Here's how the part is built. I have some questions about the finished solid (model axes, mm). A direction names the side the tool comes from. Coordinates: 2 decimals unless noted, no trailing zeros. Loops run counter-clockwise (first coordinate to the right, second up) from the corner with the lowest first, then second, coordinate; pieces in that order, holes last.
from build123d import *

# Parameters (mm, degrees)
F0_R     = 6.7
F0_R_2   = 4.1
F1_DEPTH = 2
F2_R     = 6.2
F2_R_2   = 4.1
F3_DEPTH = 10
F4_SIZE  = 0.5


with BuildPart() as f1:
    # F0 (on Top) → F1 (new body)
    with BuildSketch(Plane.XY):
        Circle(F0_R)
        Circle(F0_R_2, mode=Mode.SUBTRACT)
    extrude(amount=F1_DEPTH)

    # F2 (on face) → F3 (join)
    with BuildSketch(Plane.XY.offset(2)):
        Circle(F2_R)
        Circle(F2_R_2, mode=Mode.SUBTRACT)
    extrude(amount=F3_DEPTH)

    # F4
    f4_edges = [f1.edges().sort_by_distance(p)[0] for p in [
        (-4.1, 0, 12),
        (-6.2, 0, 12),
    ]]
    chamfer(f4_edges, length=F4_SIZE)


solid = f1.part
Q1. Will these pins go through, and if not, where does the flat tip stop? P1, Ø2, axis at x = -5, z = 6, coming from the +Y side; P2, Ø1, axis at y = 3.5, z = 8, coming from the -X side; P3, Ø5, axis at y = -0.5, z = 9, coming from the +X side.
Q2. We'd pull the mould along Y, two halves only. Please class faces 3 (the cylindrical face through (-0.534, 4.065, 5.67)), 4 (the cylindrical face through (-6.694, 0.295, 0.986)), 5 (the flat face through (-4, 3, 12)): pulls with the +Y half, pulls with the -Y half, needs draft (parallel to the pull), parting line crosses it, or undercut.
Q3. Please list where these lines run through material, in increasing order: probe 1 along Y at (x, z) = (0, 5.25); probe 2 along X at (y, z) = (2.25, 11); probe 3 along X at (y, z) = (3.5, 10).
Q4. Suppose I cut it at C-C on z = 5. Write out the boundary of the cut face in (x, y).
Q5. For faces 1 (the cylindrical face through (2.86, -5.5, 6.68)), 2 (the flat face through (-0.1, -4.4, 0)), which set-ups out of +Z, -Z, +X, -X, +Y, -Y let a thin tool reach every point of the face, with its end or its side?
Q6. Suppose I cut it at A-A on y = 0. Write out the boundary of the cut face in (x, z).
Check values:
1. P1: stops at y = 4.74
1. P2: stops at x = -5.43
1. P3: stops at x = 6.2
2. face 3: undercut
2. face 4: parting line crosses it
2. face 5: needs draft
3. probe 1: y = -6.2 to -4.1, 4.1 to 6.2
3. probe 2: x = -5.78 to -3.43, 3.43 to 5.78
3. probe 3: x = -5.12 to -2.14, 2.14 to 5.12
4. outline: circle Ø12.4 at (0, 0); hole circle Ø8.2 at (0, 0)
5. face 1: +Z
5. face 2: -Z, +X, -X, +Y, -Y
6. outline: (-6.7, 0) - (-4.1, 0) - (-4.1, 11.5) - (-4.6, 12) - (-5.7, 12) - (-6.2, 11.5) - (-6.2, 2) - (-6.7, 2) - close; (4.1, 0) - (6.7, 0) - (6.7, 2) - (6.2, 2) - (6.2, 11.5) - (5.7, 12) - (4.6, 12) - (4.1, 11.5) - close
